```python
from build123d import *

# Parameters (mm, degrees)
SKETCH_1_W          = 29
SKETCH_1_H          = 13.5
EXTRUDE_1_DEPTH     = 25.5
FILLET_1_R          = 0.5
SKETCH_2_W          = 4
SKETCH_2_H          = 2
CUT_EXTRUDE_1_DEPTH = 1
SKETCH_3_W          = 0.5
SKETCH_3_H          = 1
EXTRUDE_2_DEPTH     = 4
FILLET_2_R          = 0.05


with BuildPart() as part:
    # Эскиз1 → Бобышка-Вытянуть1 (new body)
    with BuildSketch(Plane.XY):
        Rectangle(SKETCH_1_W, SKETCH_1_H)
    extrude(amount=EXTRUDE_1_DEPTH)

    # Скругление1
    fillet_1_edges = [part.edges().sort_by_distance(p)[0] for p in [
        (-14.5, 0, 25.5),
        (0, -6.75, 25.5),
        (14.5, 0, 25.5),
        (0, 6.75, 25.5),
        (14.5, -6.75, 12.75),
        (-14.5, -6.75, 12.75),
        (-14.5, 6.75, 12.75),
        (14.5, 6.75, 12.75),
    ]]
    fillet(fillet_1_edges, radius=FILLET_1_R)

    # Эскиз2 → Вырез-Вытянуть1 (cut)
    with BuildSketch(Plane.XY.offset(25.5)):
        with Locations((-12.5, 0.002144421)):
            Rectangle(SKETCH_2_W, SKETCH_2_H)
    extrude(amount=-CUT_EXTRUDE_1_DEPTH, mode=Mode.SUBTRACT)

    # Эскиз3 → Бобышка-Вытянуть2 (add)
    with BuildSketch(Plane(origin=(0, 0, 0), x_dir=(-1, 0, 0), z_dir=(0, 0, -1))):
        with Locations((12.5, -3.75)):
            Rectangle(SKETCH_3_W, SKETCH_3_H)
        with Locations((-2.5, -3.75)):
            Rectangle(SKETCH_3_W, SKETCH_3_H)
        with Locations((-7.5, -3.75)):
            Rectangle(SKETCH_3_W, SKETCH_3_H)
        with Locations((-12.5, -3.75)):
            Rectangle(SKETCH_3_W, SKETCH_3_H)
        with Locations((-12.5, 3.75)):
            Rectangle(SKETCH_3_W, SKETCH_3_H)
        with Locations((-7.5, 3.75)):
            Rectangle(SKETCH_3_W, SKETCH_3_H)
        with Locations((-2.5, 3.75)):
            Rectangle(SKETCH_3_W, SKETCH_3_H)
        with Locations((12.5, 3.75)):
            Rectangle(SKETCH_3_W, SKETCH_3_H)
    extrude(amount=EXTRUDE_2_DEPTH)

    # Скругление2
    fillet_2_edges = [part.edges().sort_by_distance(p)[0] for p in [
        (12.25, 3.25, -2),
        (12.25, 4.25, -2),
        (12.75, 4.25, -2),
        (12.75, 3.25, -2),
        (7.25, 3.25, -2),
        (7.25, 4.25, -2),
        (7.75, 4.25, -2),
        (7.75, 3.25, -2),
        (2.25, 3.25, -2),
        (2.25, 4.25, -2),
        (2.75, 4.25, -2),
        (2.75, 3.25, -2),
        (-12.75, 3.25, -2),
        (-12.75, 4.25, -2),
        (-12.25, 4.25, -2),
        (-12.25, 3.25, -2),
        (-12.25, -3.25, -2),
        (-12.25, -4.25, -2),
        (-12.75, -4.25, -2),
        (-12.75, -3.25, -2),
        (2.75, -3.25, -2),
        (2.75, -4.25, -2),
        (2.25, -4.25, -2),
        (2.25, -3.25, -2),
        (7.75, -3.25, -2),
        (7.75, -4.25, -2),
        (7.25, -4.25, -2),
        (7.25, -3.25, -2),
        (12.75, -3.25, -2),
        (12.75, -4.25, -2),
        (12.25, -4.25, -2),
        (12.25, -3.25, -2),
    ]]
    fillet(fillet_2_edges, radius=FILLET_2_R)


solid = part.part
```
Work out the finished part from the listing and answer in its coordinate system (mm). A direction names the side the tool comes from. Give positions to 0.01 mm unless a question says otherwise; leave off trailing zeros. Loops run counter-clockwise (first coordinate to the right, second up) from the corner with the lowest first, then second, coordinate; pieces in that order, holes last. Notation, with made-up numbers: (4.25, 42.5) - (11.25, 42.5) arc R6 cw to (11.25, 48.5) - close; hole circle Ø6 at (-23.75, 59). An arc over 180 degrees is marked (long way). Use CSV: the item, a comma, the result in double quotes. Start each with the question number.
(1) Each of these flat-tipped pins is pushed along its axis until it touches: pin 1 (8 mm diameter, centred on x = 1.5, y = -1, fed in from -Z); pin 2 (0.7 mm diameter, centred on y = -4, z = -1.5, fed in from +X). Where does it stop, or does it pass through?
(2) Determine the mould class of faces 1 (the face through (-13, -0.998, 25)), 2 (the face through (7.25, -4, -2)), 3 (the face through (0, -6.75, 12)) for opening direction Y: released by +Y, released by -Y, zero draft, split by the parting line, or undercut.
(3) Find section B-B, the plane x = -11.25. Determine the outline of the cut face in (y, z), plus the area to 3 significant figures.
(4) Find section C-C, the plane z = -2. Count the separate pieces of the cut face and the enclosed holes in it, plus the area to 3 significant figures.
(5) Find section A-A, the plane y = 0. Determine the outline of the cut face in (x, z), plus the area to 3 significant figures.
(6) Find the intervals of material crossed by L1, parallel to Z at x = 10.5, y = -0.75; L2, parallel to Z at x = -11.25, y = 0.5, in increasing order.
(7) Find section D-D, the plane y = -4.75. Determine the outline of the cut face in (x, z), plus the area to 3 significant figures.
(8) A tool of negligible diameter and unlimited length cuts with its end or side. For faces 4 (the face through (-10.5, 0, 25)), 5 (the face through (0, 0, 25.5)), 6 (the face through (2.75, -4, -2)), 7 (the face through (12.75, 4, -2)), 8 (the face through (-12.75, -4, -2)), from which of +Z, -Z, +X, -X, +Y, -Y can it reach the whole face along a straight path? Write none if from no direction.
Results found:
1,pin 1,"z = -4"
1,pin 2,"x = 12.75"
2,face 1,"undercut"
2,face 2,"zero draft"
2,face 3,"released by -Y"
3,outline,"(-6.75, 0) - (6.75, 0) - (6.75, 25) arc R0.5 ccw to (6.25, 25.5) - (1, 25.5) - (1, 24.5) - (-1, 24.5) - (-1, 25.5) - (-6.25, 25.5) arc R0.5 ccw to (-6.75, 25) - close"
3,area,"342 mm^2"
4,separate pieces,"8"
4,enclosed holes,"0"
4,area,"3.98 mm^2"
5,outline,"(-14.5, 0) - (14.5, 0) - (14.5, 25) arc R0.5 ccw to (14, 25.5) - (-10.5, 25.5) - (-10.5, 24.5) - (-14.5, 24.5) - close"
5,area,"735 mm^2"
6,L1,"0 to 25.5"
6,L2,"0 to 24.5"
7,outline,"(-14.5, 0) - (14.5, 0) - (14.5, 25) arc R0.5 ccw to (14, 25.5) - (-14, 25.5) arc R0.5 ccw to (-14.5, 25) - close"
7,area,"739 mm^2"
8,face 4,"+Z, -X"
8,face 5,"+Z, +X, -X, +Y, -Y"
8,face 6,"-Z, +Y, -Y"
8,face 7,"-Z, +X, +Y, -Y"
8,face 8,"-Z, -X, +Y, -Y"
